from build123d import *

# Parameters (mm, degrees)
F0_W     = 170
F0_H     = 30
F1_DEPTH = 13
F3_DEPTH = 28
F4_W     = 130
F4_H     = 2
F5_DEPTH = 5
F6_SIZE  = 5
F7_R     = 5
F8_SIZE  = 1
F9_R     = 1.99999


# Not quite as in the source:
# - a fillet or chamfer is up to 0.001 mm smaller than in the source, because OpenCascade refuses the exact size


with BuildPart() as f1:
    # F0 (on Front) → F1 (new body)
    with BuildSketch(Plane.XZ):
        with Locations((0, 15)):
            Rectangle(F0_W, F0_H)
    extrude(amount=F1_DEPTH)

    # F2 (on face) → F3 (cut)
    with BuildSketch(Plane.XY.offset(30)):
        Polygon((-65, -2), (-81, -2), (-81, -12), (-75, -12), (-75, -13), (75, -13), (75, -12), (81, -12), (81, -2), (65, -2), (65, 0), (-65, 0), align=None)
    extrude(amount=-F3_DEPTH, mode=Mode.SUBTRACT)

    # F4 (on face) → F5 (join)
    with BuildSketch(Plane.XY.offset(2)):
        with Locations((0, -1)):
            Rectangle(F4_W, F4_H)
    extrude(amount=F5_DEPTH)

    # F6
    f6_edges = [f1.edges().sort_by_distance(p)[0] for p in [
        (85, -6.5, 0),
        (-85, -6.5, 0),
    ]]
    chamfer(f6_edges, length=F6_SIZE)

    # F7
    f7_edges = [f1.edges().sort_by_distance(p)[0] for p in [
        (-81, -7, 2),
        (81, -7, 2),
    ]]
    fillet(f7_edges, radius=F7_R)

    # F8
    f8_edges = [f1.edges().sort_by_distance(p)[0] for p in [
        (0, -13, 0),
        (0, 0, 0),
    ]]
    chamfer(f8_edges, length=F8_SIZE)

    # F9 (radius 2 in the source; OpenCascade refuses exactly that, so slightly less here)
    f9_edges = [f1.edges().sort_by_distance(p)[0] for p in [
        (-85, -6.5, 5),
        (-85, -6.5, 30),
        (-81, -7, 30),
        (81, -7, 30),
        (85, -6.5, 30),
        (85, -6.5, 5),
        (65, -1, 7),
        (65, -1, 30),
        (75, -12.5, 2),
        (75, -12.5, 30),
        (-65, -1, 30),
        (-65, -1, 7),
        (-75, -12.5, 2),
        (-75, -12.5, 30),
        (85, 0, 17.5),
        (83, 0, 3),
        (83, -13, 3),
        (85, -13, 17.5),
        (-85, 0, 17.5),
        (-83, 0, 3),
        (-85, -13, 17.5),
        (-83, -13, 3),
    ]]
    fillet(f9_edges, radius=F9_R)


solid = f1.part
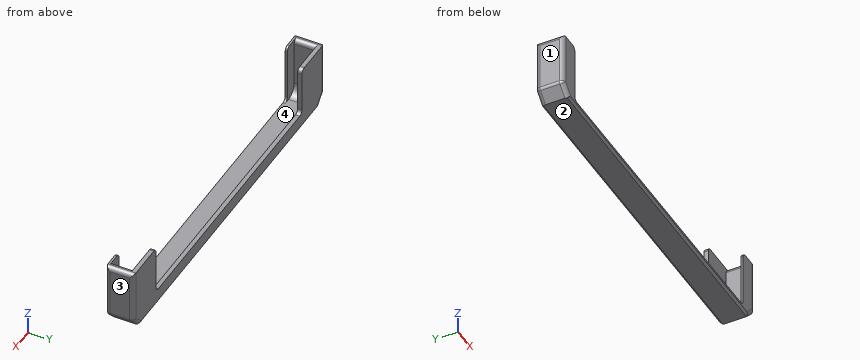
Geometry: final body of the model. Coordinates: model frame, mm. Face numbers are marked on the shaded views. Give positions to 0.01 mm unless a question says otherwise; leave off trailing zeros. Order: outer loops, then holes, each group sorted by start corner. A loop starts at its lowest first (then second) coordinate and runs counter-clockwise, first axis right, second up. Notation, with made-up numbers: (-4.5, 49.5) -> (54.5, 49.5) arc R17 cw to (54.5, 62.5) -> close; hole circle Ø4 at (-10.5, -17.75). An arc over 180 degrees is marked (long way). Put each result on its own line as item: value.
Q1. Draft query along X for the marked faces 1, 2, 3 and 4. Return one class per face: released by +X, released by -X, zero draft, split by the parting line, or undercut.
Here are the results:
face 1: released by -X
face 2: zero draft
face 3: released by +X
face 4: undercut
Q2. Pin query (flat end, axial travel): pin 1 (1.1 mm diameter, centred on y = -12.5, z = 15, fed in from +X); pin 2 (3 mm diameter, centred on x = 14.5, y = -1.5, fed in from +Z); pin 3 (0.5 mm diameter, centred on y = -12.5, z = 21.5, fed in from -X). Return the tip coordinate at first contact, or that it passes through.
Here are the results:
pin 1: stops at x = 84.76
pin 2: stops at z = 7
pin 3: stops at x = -84.56
Q3. Material intervals for L1, parallel to X at y = -3.5, z = 10; L2, parallel to Z at x = 53.5, y = -2.5; L3, parallel to Y at x = -68.5, z = 28.5, sorted ascending.
Here are the results:
L1: x = -85 to -81, 81 to 85
L2: z = 0 to 2
L3: y = -2 to 0
Q4. Section B-B, the plane x = -10.5. Return loops of the section in (y, z), then the cut area to 3 significant figures.
Here are the results:
outline: (-13, 1) -> (-12, 0) -> (-1, 0) -> (0, 1) -> (0, 7) -> (-2, 7) -> (-2, 2) -> (-13, 2) -> close
area: 35.0 mm^2
Q5. Section A-A, the plane z = 11.5. Return loops of the section in (x, y), then the cut area to 3 significant figures.
Here are the results:
outline: (-85, -11) arc R2 ccw to (-83, -13) -> (-75, -13) -> (-75, -12) -> (-81, -12) -> (-81, -2) -> (-65, -2) -> (-65, 0) -> (-83, 0) arc R2 ccw to (-85, -2) -> close; (65, -2) -> (81, -2) -> (81, -12) -> (75, -12) -> (75, -13) -> (83, -13) arc R2 ccw to (85, -11) -> (85, -2) arc R2 ccw to (83, 0) -> (65, 0) -> close
area: 177 mm^2
